```python
from build123d import *

# Parameters (mm, degrees)
F1_DEPTH  = 19.05
F2_W      = 25.4
F2_H      = 25.4
F3_DEPTH  = 25.4
F4_R      = 14.3990784814
F1_FACE_W = 25.4
F1_FACE_H = 25.4
F5_DEPTH  = 25.4


with BuildPart() as f1:
    # F0 (on Front) → F1 (new body)
    with BuildSketch(Plane.XZ):
        Polygon((76.2624083042, 0), (74.8843400498, 76.1875378778), (-71.1656599502, 76.1875378778), (-69.7875916958, 0), align=None)
    extrude(amount=F1_DEPTH)

    # F2 (on face) → F3 (cut)
    with BuildSketch(Plane.XZ.offset(19.05)):
        with Locations((-31.1477660805, 46.7091660619)):
            Rectangle(F2_W, F2_H)
    extrude(amount=-F3_DEPTH, mode=Mode.SUBTRACT)

    # F4 (on face) + F1_face (on face) → F5 (cut)
    with BuildSketch(Plane(origin=(0, 0, 0), x_dir=(-1, 0, 0), z_dir=(0, 1, 0))):
        with Locations((-36.9891412556, 42.8554788232)):
            Circle(F4_R)
    with BuildSketch(Plane(origin=(2.548374177, -19.05, 38.0937689389), x_dir=(1, 0, 0), z_dir=(0, -1, 0))):
        Polygon((-73.7140341272, 38.0937689389), (-72.3359658728, -38.0937689389), (73.7140341272, -38.0937689389), (72.3359658728, 38.0937689389), align=None)
        with Locations((-33.6961402575, 8.615397123)):
            Rectangle(F1_FACE_W, F1_FACE_H, mode=Mode.SUBTRACT)
    extrude(amount=-F5_DEPTH, dir=(0, 1, 0), mode=Mode.SUBTRACT)


solid = f1.part
```
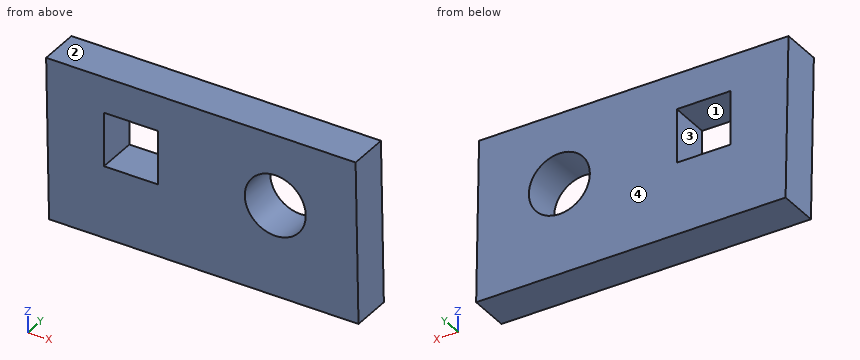
Here's how the part is built. I have some questions about the finished solid (model axes, mm). Face numbers are marked on the shaded views. A direction names the side the tool comes from. Coordinates: 2 decimals unless noted, no trailing zeros. Order: outer loops, then holes, each group sorted by start corner. A loop starts at its lowest first (then second) coordinate and runs counter-clockwise, first axis right, second up. Notation, with made-up numbers: (-19.75, 29) - (14.25, 29) arc R8 ccw to (14.25, 35) - close; hole circle Ø11 at (77, 86.5). An arc over 180 degrees is marked (long way). One line per question, with ' | ' between items. Start each with the question number.
1. If we section it at C-C (y = -9.5): Write out the boundary of the cut face in (x, z).
2. If we section it at D-D (x = 31.5): Write out the boundary of the cut face in (y, z), and give its area (3 significant figures).
3. Please list where these lines run through material, in increasing order: line 1 along X through (y, z) = (-17.75, 41.5); line 2 along X through (y, z) = (-13.5, 49); line 3 along Z through (x, y) = (-41.5, -16.25). Write a range as [from, to].
4. If we section it at A-A (x = -20): Write out the boundary of the cut face in (y, z).
5. If we section it at B-B (z = 44.5): Write out the boundary of the cut face in (x, y).
6. Which directions (+Z, -Z, +X, -X, +Y, -Y) give clear straight access to the entire face, cutting with the end or side of a thin tool? Please do the marked faces 3 and 4.
7. I'm going to push flat-ended pins straight in: pin 1 Ø4 at (y, z) = (-16, 45) entering from -X; pin 2 Ø10 at (y, z) = (-6, 17) entering from -X; pin 3 Ø17.5 at (x, z) = (36.99, 42.86) entering from +Y. Where does each tip first touch, or does it pass through?
8. If we mould it in two halves opening along X, with no side actions, what happens to the marked faces 1 and 2? For each: released by +X, released by -X, zero draft, split by the parting line, or undercut.
Model answer:
1) outline: (-71.17, 76.19) - (-69.79, 0) - (76.26, 0) - (74.88, 76.19) - close; hole (-43.85, 34.01) - (-18.45, 34.01) - (-18.45, 59.41) - (-43.85, 59.41) - close; hole circle Ø28.8 at (36.99, 42.86)
2) outline: (-19.05, 0) - (0, 0) - (0, 29.54) - (-19.05, 29.54) - close; (-19.05, 56.17) - (0, 56.17) - (0, 76.19) - (-19.05, 76.19) - close | area: 944 mm²
3) line 1: x = [-70.54, -43.85], [-18.45, 22.65], [51.32, 75.51] | line 2: x = [-70.67, -43.85], [-18.45, 23.97], [50.01, 75.38] | line 3: z = [0, 34.01], [59.41, 76.19]
4) outline: (-19.05, 0) - (0, 0) - (0, 34.01) - (-19.05, 34.01) - close; (-19.05, 59.41) - (0, 59.41) - (0, 76.19) - (-19.05, 76.19) - close
5) outline: (-70.59, -19.05) - (-43.85, -19.05) - (-43.85, 0) - (-70.59, 0) - close; (-18.45, -19.05) - (22.68, -19.05) - (22.68, 0) - (-18.45, 0) - close; (51.29, -19.05) - (75.46, -19.05) - (75.46, 0) - (51.29, 0) - close
6) face 3: +Y, -Y | face 4: +Z, -Z, +X, -X, +Y
7) pin 1: stops at x = -70.64 | pin 2: stops at x = -70.19 | pin 3: passes through
8) face 1: undercut | face 2: zero draft
